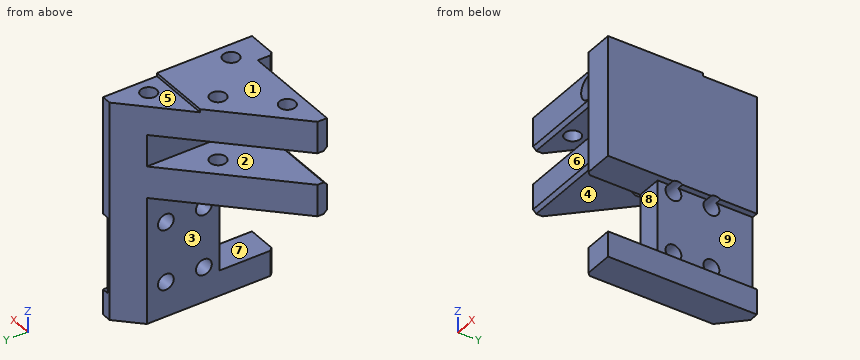
```python
from build123d import *

# Parameters (mm, degrees)
EXTRUDE_1_DEPTH      = 70
SKETCH_2_W           = 45.532219889
SKETCH_2_H           = 5
CUT_EXTRUDE_1_DEPTH  = 100.498743711
SKETCH_3_W           = 35
SKETCH_3_H           = 10
SKETCH_3_H_2         = 46.866381138
CUT_EXTRUDE_2_DEPTH  = 98.082439195
CUT_EXTRUDE_3_DEPTH  = 100.498743711
CUT_EXTRUDE_7_REACH  = 101.499
SKETCH_9_R           = 2.5
CHAMFER_1_SIZE       = 1
SKETCH_11_R          = 3.75
CUT_EXTRUDE_10_DEPTH = 8
CUT_EXTRUDE_11_DEPTH = 100.498743711
CUT_EXTRUDE_12_DEPTH = 1
SKETCH_15_W          = 24
SKETCH_15_H          = 17
CUT_EXTRUDE_14_DEPTH = 10
SKETCH_16_R          = 2.5
CUT_EXTRUDE_15_DEPTH = 91.183146984
SKETCH_17_W          = 24
SKETCH_17_H          = 30
CUT_EXTRUDE_16_DEPTH = 2
SKETCH_7_R           = 2.5
CUT_EXTRUDE_17_DEPTH = 80.429213769
CHAMFER_2_SIZE       = 1
CHAMFER_3_SIZE       = 1


with BuildPart() as part:
    # 草图1 → 拉伸1 (new body)
    with BuildSketch(Plane.XY):
        Polygon((0, 0), (50, 0), (50, 50), align=None)
    extrude(amount=EXTRUDE_1_DEPTH)

    # 草图2 → 切除-拉伸1 (cut, through all)
    with BuildSketch(Plane.XY.offset(70)):
        with Locations((17.233890055, 2.5)):
            Rectangle(SKETCH_2_W, SKETCH_2_H)
    extrude(amount=-CUT_EXTRUDE_1_DEPTH, mode=Mode.SUBTRACT)

    # 草图3 → 切除-拉伸2 (cut, through all)
    with BuildSketch(Plane.XZ.offset(-5)):
        with Locations((22.5, 55)):
            Rectangle(SKETCH_3_W, SKETCH_3_H)
        with Locations((22.5, 16.566809431)):
            Rectangle(SKETCH_3_W, SKETCH_3_H_2)
    extrude(amount=-CUT_EXTRUDE_2_DEPTH, mode=Mode.SUBTRACT)

    # 草图4 → 切除-拉伸3 (cut, through all)
    with BuildSketch(Plane.XY.offset(70)):
        Polygon((5, 5), (8, 5), (8, 8), align=None)
    extrude(amount=-CUT_EXTRUDE_3_DEPTH, mode=Mode.SUBTRACT)

    # 切除-拉伸7: up to this face of the body (flat: up to its plane)
    cut_extrude_7_end = Plane(part.part.faces().sort_by_distance((28.49122807, 16.745614035, 50))[0])
    # 草图9 → 切除-拉伸7 (cut, up to the picked face)
    with BuildSketch(Plane.XY.offset(70), mode=Mode.PRIVATE) as cut_extrude_7_sk1:
        with Locations((45, 36)):
            Circle(SKETCH_9_R)
    cut_extrude_7_tool1 = split(extrude(cut_extrude_7_sk1.sketch, amount=-CUT_EXTRUDE_7_REACH, mode=Mode.PRIVATE), bisect_by=cut_extrude_7_end, keep=Keep.BOTH, mode=Mode.PRIVATE)
    # 草图9 → 切除-拉伸7 (cut, up to the picked face)
    with BuildSketch(Plane.XY.offset(70), mode=Mode.PRIVATE) as cut_extrude_7_sk2:
        with Locations((45, 10)):
            Circle(SKETCH_9_R)
    cut_extrude_7_tool2 = split(extrude(cut_extrude_7_sk2.sketch, amount=-CUT_EXTRUDE_7_REACH, mode=Mode.PRIVATE), bisect_by=cut_extrude_7_end, keep=Keep.BOTH, mode=Mode.PRIVATE)
    # 草图9 → 切除-拉伸7 (cut, up to the picked face)
    with BuildSketch(Plane.XY.offset(70), mode=Mode.PRIVATE) as cut_extrude_7_sk3:
        with Locations((19, 10)):
            Circle(SKETCH_9_R)
    cut_extrude_7_tool3 = split(extrude(cut_extrude_7_sk3.sketch, amount=-CUT_EXTRUDE_7_REACH, mode=Mode.PRIVATE), bisect_by=cut_extrude_7_end, keep=Keep.BOTH, mode=Mode.PRIVATE)
    add(cut_extrude_7_tool1.solids().sort_by(Axis((45, 36, 70), (0, 0, -1)))[0], mode=Mode.SUBTRACT)
    add(cut_extrude_7_tool2.solids().sort_by(Axis((45, 10, 70), (0, 0, -1)))[0], mode=Mode.SUBTRACT)
    add(cut_extrude_7_tool3.solids().sort_by(Axis((19, 10, 70), (0, 0, -1)))[0], mode=Mode.SUBTRACT)

    # 倒角1
    chamfer_1_edges = [part.edges().sort_by_distance(p)[0] for p in [
        (24, 5, 60),
        (24, 5, 40),
        (24, 5, 50),
    ]]
    chamfer(chamfer_1_edges, length=CHAMFER_1_SIZE)

    # 草图11 → 切除-拉伸10 (cut)
    with BuildSketch(Plane.XZ.offset(-5)):
        with Locations((34, 65)):
            Circle(SKETCH_11_R)
    extrude(amount=-CUT_EXTRUDE_10_DEPTH, mode=Mode.SUBTRACT)

    # 草图13 → 切除-拉伸11 (cut, through all)
    with BuildSketch(Plane.XY.offset(70)):
        Polygon((50, 50), (47, 47), (50, 47), align=None)
    extrude(amount=-CUT_EXTRUDE_11_DEPTH, mode=Mode.SUBTRACT)

    # 草图14 → 切除-拉伸12 (cut)
    with BuildSketch(Plane.XY.offset(70)):
        Polygon((50, 47), (47, 47), (30, 30), (50, 30), align=None)
    extrude(amount=-CUT_EXTRUDE_12_DEPTH, mode=Mode.SUBTRACT)

    # 草图15 → 切除-拉伸14 (cut)
    with BuildSketch(Plane.ZY.offset(-40)):
        with Locations((20, 8.5)):
            Rectangle(SKETCH_15_W, SKETCH_15_H)
    extrude(amount=-CUT_EXTRUDE_14_DEPTH, mode=Mode.SUBTRACT)

    # 草图16 → 切除-拉伸15 (cut, through all)
    with BuildSketch(Plane.ZY.offset(-40)):
        with Locations((30, 34)):
            Circle(SKETCH_16_R)
        with Locations((30, 22)):
            Circle(SKETCH_16_R)
        with Locations((11, 34)):
            Circle(SKETCH_16_R)
        with Locations((11, 22)):
            Circle(SKETCH_16_R)
    extrude(amount=-CUT_EXTRUDE_15_DEPTH, mode=Mode.SUBTRACT)

    # 草图17 → 切除-拉伸16 (cut)
    with BuildSketch(Plane(origin=(50, 0, 0), x_dir=(0, 0, -1), z_dir=(1, 0, 0))):
        with Locations((-20, 32)):
            Rectangle(SKETCH_17_W, SKETCH_17_H)
    extrude(amount=-CUT_EXTRUDE_16_DEPTH, mode=Mode.SUBTRACT)

    # 草图7 → 切除-拉伸17 (cut, through all)
    with BuildSketch(Plane(origin=(0, 0, 40), x_dir=(-1, 0, 0), z_dir=(0, 0, -1))):
        with Locations((-32.036330274, 22.963669726)):
            Circle(SKETCH_7_R)
    extrude(amount=-CUT_EXTRUDE_17_DEPTH, mode=Mode.SUBTRACT)

    # 倒角2
    chamfer_2_edges = [part.edges().sort_by_distance(p)[0] for p in [
        (40, 0, 51),
    ]]
    chamfer(chamfer_2_edges, length=CHAMFER_2_SIZE)

    # 倒角3
    chamfer_3_edges = [part.edges().sort_by_distance(p)[0] for p in [
        (40, 0, 4),
    ]]
    chamfer(chamfer_3_edges, length=CHAMFER_3_SIZE)


solid = part.part
```
For this review, take the finished solid that the model builds, in its own axes (mm). Face numbers are marked on the shaded views. A direction names the side the tool comes from. Coordinates: 2 decimals unless noted, no trailing zeros. Loops run counter-clockwise (first coordinate to the right, second up) from the corner with the lowest first, then second, coordinate; pieces in that order, holes last. Notation, with made-up numbers: (-16, -40) - (14, -40) arc R17 cw to (14, -14) - close; hole circle Ø9 at (75, 18.25). An arc over 180 degrees is marked (long way). Use one line per item in the form item = value. Start each with the question number.
1) Draft analysis for pull direction Z (two halves, no side actions). For the marked faces 1, 2, 3 and 4, state which applies: released by +Z, released by -Z, zero draft, split by the parting line, or undercut.
2) For the marked faces 5, 6, 7, 8 and 9, list the 3-axis set-ups (+Z, -Z, +X, -X, +Y, -Y) from which the entire face can be reached by the end or side of a thin tool; tool diameter is ignored.
3) Take a section at A-A (y = 10). State the section outline as (x, z) points.
4) Take a section at B-B (x = 24). State the section outline as (y, z) points.
5) Take a section at C-C (z = 11). State the section outline as (x, y) points, plus the area to 4 significant figures.
6) Take a section at D-D (x = 43.5). State the section outline as (y, z) points, plus the area to 3 significant figures.
7) To check wall thickness, follow probe 1 along Z at (x, y) = (23, 20.5); probe 2 along Y at (x, z) = (46.5, 30); probe 3 along Y at (x, z) = (40.5, 12). State the ranges of each line that lie inside material, in increasing order. Write a range as from..to.
8) For pin 1 (6 mm diameter, centred on x = 34.5, z = 63.5, fed in from -Y); pin 2 (8 mm diameter, centred on x = 36.5, y = 41.5, fed in from +Z); pin 3 (10 mm diameter, centred on x = 34.5, y = 9, fed in from -Z), all flat-tipped, find the tip position at first contact; note any pin that passes through.
From the geometry:
q1.face_1 = released by +Z
q1.face_2 = undercut
q1.face_3 = undercut
q1.face_4 = released by -Z
q2.face_5 = +Z, +X, -X, +Y
q2.face_6 = +Z, -Z, -X, -Y
q2.face_7 = +X, -Y
q2.face_8 = +X, -X, -Y
q2.face_9 = +X, +Y, -Y
q3.outline = (10, 40) - (40, 40) - (40, 32) - (50, 32) - (50, 70) - (47.5, 70) - (47.5, 50) - (42.5, 50) - (42.5, 70) - (21.5, 70) - (21.5, 60) - (40, 60) - (40, 50) - (10, 50) - close; (10, 60) - (16.5, 60) - (16.5, 70) - (10, 70) - close; (40, 0) - (50, 0) - (50, 8) - (40, 8) - close; hole circle Ø7.5 at (34, 65)
q4.outline = (5, 41) - (6, 40) - (24, 40) - (24, 50) - (6, 50) - (5, 49) - close; (5, 61) - (6, 60) - (24, 60) - (24, 70) - (5, 70) - close
q5.outline = (40, 17) - (48, 17) - (48, 19.5) - (40, 19.5) - close; (40, 24.5) - (48, 24.5) - (48, 31.5) - (40, 31.5) - close; (40, 36.5) - (48, 36.5) - (48, 47) - (47, 47) - (40, 40) - close
q5.area = 135.5 mm2
q6.outline = (0, 0) - (43.5, 0) - (43.5, 69) - (38, 69) - (38, 50) - (34, 50) - (34, 69) - (30, 69) - (30, 70) - (12, 70) - (12, 50) - (8, 50) - (8, 70) - (0, 70) - (0, 32) - (17, 32) - (17, 8) - (0, 8) - close; hole circle Ø5 at (22, 11); hole circle Ø5 at (22, 30); hole circle Ø5 at (34, 11); hole circle Ø5 at (34, 30)
q6.area = 2,390 mm2
q7.probe_1 = 40..50, 60..70
q7.probe_2 = 17..19.5, 24.5..31.5, 36.5..46.5
q7.probe_3 = 17..19.71, 24.29..31.71, 36.29..40.5
q8.pin_1 = 5
q8.pin_2 = 69
q8.pin_3 = 40
